Read the model definition and answer for the solid it produces. Units are mm, in the model's axes. Face numbers are marked on the shaded views. A direction names the side the tool comes from. Give positions to 0.01 mm unless a question says otherwise; leave off trailing zeros. Loops run counter-clockwise (first coordinate to the right, second up) from the corner with the lowest first, then second, coordinate; pieces in that order, holes last. Notation, with made-up numbers: (22.25, -8) - (32.25, -8) arc R16 cw to (32.25, 20) - close; hole circle Ø9 at (-22, 52.25). An arc over 180 degrees is marked (long way). Put each result on its own line as item: value. Start each with the question number.
1. A cutting plane is placed at C-C, the plane x = 41. Determine the outline of the cut face in (y, z).
2. A cutting plane is placed at B-B, the plane z = 6.35. Determine the outline of the cut face in (x, y), plus the area to 3 significant figures.
3. For the marked faces 1, 2, 3 and 4, determine the directions among +Z, -Z, +X, -X, +Y, -Y from which every point of the face is accessible in a straight line to the end or side of a thin tool.
4. For a pull along X with two mould halves and no side action, classify the marked faces 5, 6 and 7 as released by +X, released by -X, zero draft, split by the parting line, or undercut.
5. Consider L1, parallel to Z at x = 54.5, y = 13; L2, parallel to X at y = -8, z = 13; L3, parallel to X at y = 26, z = 9.5. Determine where each line is inside the solid, lowest interval first. Write a range as from..to.
6. Given pin 1 Ø4.5 at (y, z) = (-0.52, 6.35) entering from +X; pin 2 Ø1.5 at (x, y) = (18.5, 21) entering from -Z; pin 3 Ø4 at (x, z) = (24.5, 5) entering from +Y; pin 4 Ø6.5 at (x, z) = (12.5, 7) entering from -Y, each flat-ended and moving along its own axis, determine where each tip first touches the part or whether it passes through.
7. A cutting plane is placed at D-D, the plane y = -1. Determine the outline of the cut face in (x, z), plus the area to 3 significant figures.
8. A cutting plane is placed at A-A, the plane x = -12. Determine the outline of the cut face in (y, z) (3 decimals), plus the area to 3 significant figures.
```python
from build123d import *

# Parameters (mm, degrees)
SKETCH1_W             = 12.7
SKETCH1_H             = 43.942
BOSS_EXTRUDE1_DEPTH   = 12.7
BOSS_EXTRUDE1_2_DEPTH = 12.7
SKETCH2_R             = 3.175
SKETCH2_R_2           = 2.54
CUT_EXTRUDE1_DEPTH    = 87.166453569
BOSS_EXTRUDE3_REACH   = 76.696
SKETCH4_W             = 12.7
SKETCH4_H             = 5.08
SKETCH5_W             = 3.81
SKETCH5_H             = 43.942
BOSS_EXTRUDE4_DEPTH   = 19.05
SKETCH6_W             = 78.994
SKETCH6_H             = 43.942
BOSS_EXTRUDE5_DEPTH   = 6.35


with BuildPart() as part:
    # Sketch1 → Boss-Extrude1 (new body)
    with BuildSketch(Plane.XY):
        with Locations((-13.235289256, 10.018305785)):
            Rectangle(SKETCH1_W, SKETCH1_H)
    extrude(amount=BOSS_EXTRUDE1_DEPTH)


with BuildPart() as body_2:
    # Sketch1 → Boss-Extrude1 2 (new body)
    with BuildSketch(Plane.XY):
        with Locations((53.058710744, 10.018305785)):
            Rectangle(SKETCH1_W, SKETCH1_H)
    extrude(amount=BOSS_EXTRUDE1_2_DEPTH)


with BuildPart() as cut_extrude1_tool:
    # Sketch2 → Cut-Extrude1 (new, through all)
    with BuildSketch(Plane.ZY.offset(19.585289256)):
        with Locations(Location((6.35, 19.289305785, 0), (0, 0, 270))):
            Circle(SKETCH2_R)
        with Locations(Location((6.35, -0.522694215, 0), (0, 0, 270))):
            Circle(SKETCH2_R_2)
    extrude(amount=-CUT_EXTRUDE1_DEPTH)


with BuildPart() as part_1:
    add(part.part)

    # Cut-Extrude1: cut by cut_extrude1_tool
    add(cut_extrude1_tool.part, mode=Mode.SUBTRACT)


with BuildPart() as body_2_1:
    add(body_2.part)

    # Cut-Extrude1: cut by cut_extrude1_tool
    add(cut_extrude1_tool.part, mode=Mode.SUBTRACT)

    # Sketch4 → Boss-Extrude3 (add, up to next)
    with BuildSketch(Plane(origin=(-6.885289256, 0, 0), x_dir=(0, 0, -1), z_dir=(1, 0, 0)), mode=Mode.PRIVATE) as boss_extrude3_sk1:
        with Locations((-6.35, 10.018305785)):
            Rectangle(SKETCH4_W, SKETCH4_H)
    boss_extrude3_tool1 = extrude(boss_extrude3_sk1.sketch, amount=BOSS_EXTRUDE3_REACH, mode=Mode.PRIVATE) - body_2_1.part

    add(part_1.part)  # Boss-Extrude3 merges part
    add(boss_extrude3_tool1.solids().sort_by_distance((-6.885289, 10.018306, 6.35))[0])

    # Sketch5 → Boss-Extrude4 (add)
    with BuildSketch(Plane.XY.offset(12.7)):
        with Locations((-17.680289256, 10.018305785)):
            Rectangle(SKETCH5_W, SKETCH5_H)
        with Locations((57.503710744, 10.018305785)):
            Rectangle(SKETCH5_W, SKETCH5_H)
    extrude(amount=BOSS_EXTRUDE4_DEPTH)

    # Sketch6 → Boss-Extrude5 (add)
    with BuildSketch(Plane.XY.offset(31.75)):
        with Locations((19.911710744, 10.018305785)):
            Rectangle(SKETCH6_W, SKETCH6_H)
    extrude(amount=BOSS_EXTRUDE5_DEPTH)


solid = body_2_1.part
```
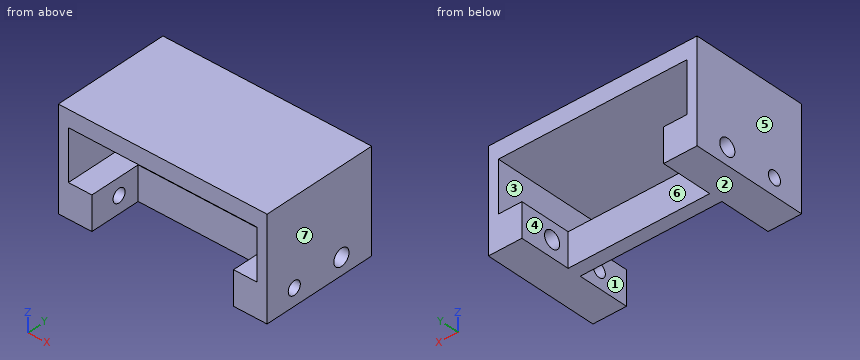
Return value:
1. outline: (-11.95, 31.75) - (31.99, 31.75) - (31.99, 38.1) - (-11.95, 38.1) - close; (7.48, 0) - (12.56, 0) - (12.56, 12.7) - (7.48, 12.7) - close
2. outline: (-19.59, -11.95) - (-6.89, -11.95) - (-6.89, -3.06) - (-19.59, -3.06) - close; (-19.59, 2.02) - (-6.89, 2.02) - (-6.89, 7.48) - (46.71, 7.48) - (46.71, 2.02) - (59.41, 2.02) - (59.41, 16.11) - (46.71, 16.11) - (46.71, 12.56) - (-6.89, 12.56) - (-6.89, 16.11) - (-19.59, 16.11) - close; (-19.59, 22.46) - (-6.89, 22.46) - (-6.89, 31.99) - (-19.59, 31.99) - close; (46.71, -11.95) - (59.41, -11.95) - (59.41, -3.06) - (46.71, -3.06) - close; (46.71, 22.46) - (59.41, 22.46) - (59.41, 31.99) - (46.71, 31.99) - close
2. area: 1,100 mm2
3. face 1: -Z, -Y
3. face 2: -Z, +X, -X, +Y, -Y
3. face 3: +Y, -Y
3. face 4: -Z, +Y
4. face 5: released by -X
4. face 6: undercut
4. face 7: released by +X
5. L1: z = 0..12.7, 31.75..38.1
5. L2: x = -19.59..-15.78, 55.6..59.41
5. L3: x = -19.59..-6.89, 46.71..59.41
6. pin 1: passes through
6. pin 2: stops at z = 31.75
6. pin 3: stops at y = 12.56
6. pin 4: stops at y = 7.48
7. outline: (-19.59, 0) - (-6.89, 0) - (-6.89, 3.86) - (-19.59, 3.86) - close; (-19.59, 8.84) - (-6.89, 8.84) - (-6.89, 12.7) - (-15.78, 12.7) - (-15.78, 31.75) - (55.6, 31.75) - (55.6, 12.7) - (46.71, 12.7) - (46.71, 8.84) - (59.41, 8.84) - (59.41, 38.1) - (-19.59, 38.1) - close; (46.71, 0) - (59.41, 0) - (59.41, 3.86) - (46.71, 3.86) - close
7. area: 843 mm2
8. outline: (-11.953, 0) - (31.989, 0) - (31.989, 12.7) - (-11.953, 12.7) - close; (-11.953, 31.75) - (31.989, 31.75) - (31.989, 38.1) - (-11.953, 38.1) - close; hole circle Ø5.08 at (-0.523, 6.35); hole circle Ø6.35 at (19.289, 6.35)
8. area: 785 mm2
